```python
from build123d import *

# Parameters (mm, degrees)
SKETCH1_R          = 9
BASE_FLANGE1_DEPTH = 4
CUT_EXTRUDE1_DEPTH = 10
SKETCH7_R          = 1.55
CUT_EXTRUDE2_DEPTH = 10


# Sheet-metal steps are written as plain solids
with BuildPart() as part:
    # Sketch1 → Base-Flange1 (new body)
    with BuildSketch(Plane(origin=(0, 0, 0), x_dir=(1, 0, 0), z_dir=(0, 1, 0))):
        with Locations(Location((0, 0, 0), (0, 0, 270))):
            Circle(SKETCH1_R)
    extrude(amount=-BASE_FLANGE1_DEPTH)

    # Sketch6 → Cut-Extrude1 (cut)
    with BuildSketch(Plane(origin=(0, 0, 0), x_dir=(1, 0, 0), z_dir=(0, 1, 0))):
        with BuildLine():
            Line((-2, 1.5), (2, 1.5))
            ThreePointArc((2, 1.5), (2.5, 0), (2, -1.5))
            Line((2, -1.5), (0, -1.5))
            Line((0, -1.5), (-2, -1.5))
            ThreePointArc((-2, -1.5), (-2.5, 0), (-2, 1.5))
        make_face()
    extrude(amount=-CUT_EXTRUDE1_DEPTH, mode=Mode.SUBTRACT)

    # Sketch7 → Cut-Extrude2 (cut)
    with BuildSketch(Plane(origin=(0, 0, 0), x_dir=(1, 0, 0), z_dir=(0, 1, 0))):
        with Locations(Location((-5.45, 0, 0), (0, 0, 270))):
            Circle(SKETCH7_R)
        with Locations(Location((5.45, 0, 0), (0, 0, 270))):
            Circle(SKETCH7_R)
    extrude(amount=-CUT_EXTRUDE2_DEPTH, mode=Mode.SUBTRACT)


solid = part.part
```
The listing builds one solid part. Answer for the finished solid, in the listing's coordinates (mm). A direction names the side the tool comes from. Give positions to 0.01 mm unless a question says otherwise; leave off trailing zeros. Loops run counter-clockwise (first coordinate to the right, second up) from the corner with the lowest first, then second, coordinate; pieces in that order, holes last. Notation, with made-up numbers: (51.25, 77) - (102.25, 77) arc R20 ccw to (102.25, 94) - close; hole circle Ø9 at (30, -19.5). An arc over 180 degrees is marked (long way). Answer as CSV lines item,"result". Start each with the question number.
Item 1: A cutting plane is placed at C-C on x = -5.45. Determine the outline of the cut face in (y, z), then the cut area to 3 significant figures.
Item 2: A cutting plane is placed at A-A on z = 0. Determine the outline of the cut face in (x, y), then the cut area to 3 significant figures.
Item 3: A cutting plane is placed at B-B on y = -3.45. Determine the outline of the cut face in (x, z).
Item 4: A cutting plane is placed at D-D on x = 5. Determine the outline of the cut face in (y, z), then the cut area to 3 significant figures.
Item 5: For faces 4 (the face through (0, -2, -1.5)), 5 (the face through (0, 0, 2)), determine the directions among +Z, -Z, +X, -X, +Y, -Y from which every point of the face is accessible in a straight line to the end or side of a thin tool.
Item 6: Each of these flat-tipped pins is pushed along its axis until it touches: pin 1 (4 mm diameter, centred on x = 5.45, z = 0, fed in from +Y); pin 2 (2 mm diameter, centred on y = -3, z = -3, fed in from +X); pin 3 (1.5 mm diameter, centred on x = 1.5, y = -1, fed in from -Z). Where does it stop, or does it pass through?
Item 7: Find the intervals of material crossed by line 1 (X direction, y = -1.35, z = 0); line 2 (Z direction, x = 0.25, y = -1.9); line 3 (X direction, y = -2.05, z = -0.5), in increasing order. Write a range as from..to.
Item 8: The mould has two halves that part along X. Classify faces 1 (the face through (2.703, -1.972, 8.584)), 2 (the face through (0, -4, 2)), 3 (the face through (-2.5, -2, 0)): +X half, -X half, draft (parallel to the pull), parting line (faces both ways), or undercut.
Found:
1,outline,"(-4, -7.16) - (0, -7.16) - (0, -1.55) - (-4, -1.55) - close; (-4, 1.55) - (0, 1.55) - (0, 7.16) - (-4, 7.16) - close"
1,area,"44.9 mm^2"
2,outline,"(-9, -4) - (-7, -4) - (-7, 0) - (-9, 0) - close; (-3.9, -4) - (-2.5, -4) - (-2.5, 0) - (-3.9, 0) - close; (2.5, -4) - (3.9, -4) - (3.9, 0) - (2.5, 0) - close; (7, -4) - (9, -4) - (9, 0) - (7, 0) - close"
2,area,"27.2 mm^2"
3,outline,"circle Ø18 at (0, 0); hole circle Ø3.1 at (-5.45, 0); hole (-2, -1.5) - (2, -1.5) arc R2.5 ccw to (2, 1.5) - (-2, 1.5) arc R2.5 ccw to start; hole circle Ø3.1 at (5.45, 0)"
4,outline,"(-4, -7.48) - (0, -7.48) - (0, -1.48) - (-4, -1.48) - close; (-4, 1.48) - (0, 1.48) - (0, 7.48) - (-4, 7.48) - close"
4,area,"48.0 mm^2"
5,face 4,"+Y, -Y"
5,face 5,"+Z, -Z, +X, -X, +Y"
6,pin 1,"stops at y = 0"
6,pin 2,"stops at x = 8.77"
6,pin 3,"stops at z = -8.97"
7,line 1,"x = -9..-7, -3.9..-2.5, 2.5..3.9, 7..9"
7,line 2,"z = -9..-1.5, 1.5..9"
7,line 3,"x = -8.99..-6.92, -3.98..-2.45, 2.45..3.98, 6.92..8.99"
8,face 1,"parting line"
8,face 2,"draft"
8,face 3,"undercut"
